from build123d import *

# Parameters (mm, degrees)
PAD002_DEPTH    = 10
SKETCH008_R     = 4.5
POCKET003_DEPTH = 4
SKETCH009_R     = 2.6
POCKET004_DEPTH = 6.001
FILLET001_R     = 1


with BuildPart() as part:
    # Sketch007 → Pad002 (new body)
    with BuildSketch(Plane.YZ):
        Polygon((-21, 17), (-17, 21), (17, 21), (21, 17), (21, -17), (17, -21), (-17, -21), (-21, -17), align=None)
    extrude(amount=PAD002_DEPTH)

    # Sketch008 (on Face9 of Pad002) → Pocket003 (cut)
    with BuildSketch(Plane(origin=(0, 0, 0), x_dir=(0, 1, 0), z_dir=(-1, 0, 0))):
        Circle(SKETCH008_R)
    extrude(amount=-POCKET003_DEPTH, mode=Mode.SUBTRACT)

    # Sketch009 (on Face12 of Pocket003) → Pocket004 (cut, through all)
    with BuildSketch(Plane(origin=(4, 0, 0), x_dir=(0, 1, 0), z_dir=(-1, 0, 0))):
        Circle(SKETCH009_R)
    extrude(amount=-POCKET004_DEPTH, mode=Mode.SUBTRACT)

    # Fillet001
    fillet001_edges = [part.edges().sort_by_distance(p)[0] for p in [
        (0, -19, 19),
        (0, -21, 0),
        (0, 0, 21),
        (0, -19, -19),
        (0, 19, 19),
        (0, 0, -21),
        (0, 21, 0),
        (0, 19, -19),
        (0, -4.5, 0),
    ]]
    fillet(fillet001_edges, radius=FILLET001_R)


solid = part.part
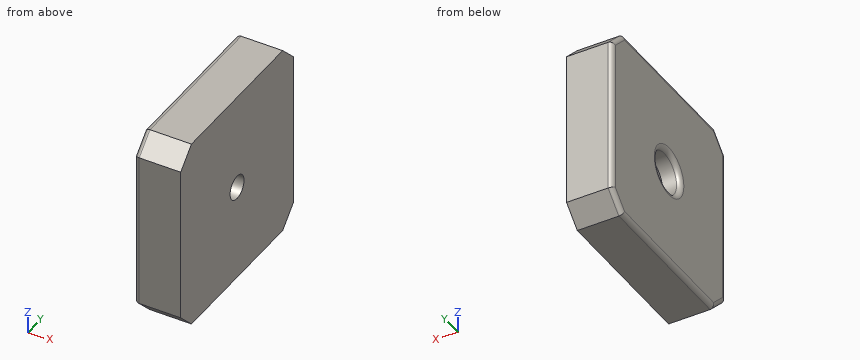
The model under review builds one solid part; all positions refer to its coordinate system, in mm. Round coordinates to 2 decimals unless told otherwise and drop trailing zeros. Order: outer loops, then holes, each group sorted by start corner. A loop starts at its lowest first (then second) coordinate and runs counter-clockwise, first axis right, second up. Notation, with made-up numbers: (39, 80.25) -> (45, 80.25) arc R35 cw to (45, 114.25) -> close; hole circle Ø6 at (77.5, 81.25). An arc over 180 degrees is marked (long way). Write item = value, one per line. Start each with the question number.
Item 1: For line 1 along Y through (x, z) = (2.35, 0); line 2 along Z through (x, y) = (8.8, 0), list the stretches that pass through material, from the lowest coordinate up.
Item 2: Consider section C-C on x = 5. Write out the cut boundary in (y, z), plus the area to 3 significant figures.
Item 3: Clearance check with a flat-ended pin moving along its axis: pin 1 Ø2.5 at (y, z) = (-2, -2) entering from -X. State where the tip first meets the part, or that it passes through.
Item 4: Consider section A-A on y = 0. Write out the cut boundary in (x, z).
Conclusion:
q1.line_1 = -21 to -4.5, 4.5 to 21
q1.line_2 = -21 to -2.6, 2.6 to 21
q2.outline = (-21, -17) -> (-17, -21) -> (17, -21) -> (21, -17) -> (21, 17) -> (17, 21) -> (-17, 21) -> (-21, 17) -> close; hole circle Ø5.2 at (0, 0)
q2.area = 1,710 mm2
q3.pin_1 = 4
q4.outline = (0, -20) arc R1 ccw to (1, -21) -> (10, -21) -> (10, -2.6) -> (4, -2.6) -> (4, -4.5) -> (1, -4.5) arc R1 ccw to (0, -5.5) -> close; (0, 5.5) arc R1 ccw to (1, 4.5) -> (4, 4.5) -> (4, 2.6) -> (10, 2.6) -> (10, 21) -> (1, 21) arc R1 ccw to (0, 20) -> close
